Source: CAD feature listing. Evaluate the final solid. Frame: model axes, mm. A direction names the side the tool comes from. Round coordinates to 2 decimals unless told otherwise and drop trailing zeros. Order: outer loops, then holes, each group sorted by start corner. A loop starts at its lowest first (then second) coordinate and runs counter-clockwise, first axis right, second up. Notation, with made-up numbers: (75.5, 57.25) - (103.5, 57.25) arc R20 cw to (103.5, 61.25) - close; hole circle Ø8 at (28, 79). An arc over 180 degrees is marked (long way). Put each result on its own line as item: value. Start each with the question number.
1) Section C-C on x = 0. Output: boundary loops of the cut face in (y, z).
2) Section D-D on z = 1.5. Output: boundary loops of the cut face in (x, y), then the cut area to 3 significant figures.
3) Section B-B on z = 5. Output: boundary loops of the cut face in (x, y).
4) Access query for faces 1 (the face through (1.7, 1.4, 4.9)), 2 (the face through (-1.7, 1.5, 4.9)), 3 (the face through (1.864, -0.314, 7.372)). Directions: +Z, -Z, +X, -X, +Y, -Y. A direction counts if a zero-diameter tool reaches every point of the face in a straight line with its end or side. Return the directions, or none.
5) Contact query for flat-ended pins moving along their axis: P1, Ø1.2, axis at x = 2.5, z = 6, coming from the +Y side; P2, Ø2, axis at y = 0, z = 4.5, coming from the +X side; P3, Ø0.6, axis at y = 1.5, z = 4.5, coming from the -X side; P4, Ø0.9, axis at y = 1.5, z = 6.5, coming from the +X side. Output: stop coordinate, or through.
6) Mould query, pull axis Z, two halves, no side actions, for faces 4 (the face through (0, -1.5, 1)), 5 (the face through (0, 0, 0)), 6 (the face through (-1.3, 0.7, 6.3)). Classes: +Z half, -Z half, draft (parallel to the pull), parting line (faces both ways), or undercut.
7) Section A-A on y = -0.75. Output: boundary loops of the cut face in (x, z).
8) Line query: probe 1 along Z at (x, y) = (-1.3, 0.3); probe 2 along Z at (x, y) = (0, 1.4); probe 3 along Y at (x, z) = (-0.95, 6.5). Output: solid intervals per line, ascending. Write a range as [from, to].
Autodesk Fusion 360 part; units mm, degrees
sketch "Sketch1" plane through (0, 0, 0) normal (0, 0, 1) x (1, 0, 0)
  line L0 (-2.85, 0.9) -> (-2.85, -1.5)
  line L1 (2.85, -1.5) -> (2.85, 0.9)
  line L2 (2.85, 0.9) -> (1.7, 0.9)
  line L3 (1.7, 0.9) -> (1.7, 2)
  line L4 (1.7, 2) -> (-1.7, 2)
  line L5 (-1.7, 2) -> (-1.7, 0.9)
  line L6 (-1.7, 0.9) -> (-2.85, 0.9)
  line L7 (-2.85, -1.5) -> (2.85, -1.5)
  dimension "d1" = 3.4
  dimension "d2" = 5.7
  dimension "d3" = 2.4
  dimension "d4" = 1.1
  dimension "d5" = 1.7
  dimension "d6" = 2
  dimension "d7" = 1.15
extrude "Extrude1" add sketch "Sketch1" along normal blind 10
sketch "Sketch2" plane through (0, -1.5, 0) normal (0, -1, 0) x (1, 0, 0)
  line L0 (-2.85, 0) -> (2.85, 0)
  line L1 (2.85, 0) -> (2.85, 10)
  line L2 (2.85, 10) -> (-2.85, 10)
  line L3 (-2.85, 10) -> (-2.85, 0)
  line L4 (1.6166, 2.2) -> (3.2332, 5)
  line L5 (3.2332, 5) -> (1.6166, 7.8)
  line L6 (1.6166, 7.8) -> (-1.6166, 7.8)
  line L7 (-1.6166, 7.8) -> (-3.2332, 5)
  line L8 (-3.2332, 5) -> (-1.6166, 2.2)
  line L9 (-1.6166, 2.2) -> (1.6166, 2.2)
  circle A0 centre (0, 5) radius 1.5
  point P0 (0, 5)
  dimension "d10" = 2.8
  dimension "d11" = 2.85
  dimension "d19" = 5
  dimension "d20" = 3
extrude "Extrude2" cut sketch "Sketch2" against normal blind 2.2 contours L1 L3 L4 L5 L6 L7 L8 L9 | A0
fillet "Fillet1" radius 0.4 4 edges at (-2.85, -0.4, 4.3363) (2.85, -0.4, 5.6637) (2.85, -0.4, 4.3363) (-2.85, -0.4, 5.6637)
fillet "Fillet2" radius 0.4 8 edges at (-1.7, 1.45, 0) (-2.85, -0.3, 0) (-2.85, -0.3, 10) (-1.7, 1.45, 10) (1.7, 1.45, 0) (2.85, -0.3, 0) (1.7, 1.45, 10) (2.85, -0.3, 10)
chamfer "Chamfer1" distance 0.2 angle 45 20 edges at (0, -1.5, 0) (2.7328, -1.5, 0.1172) (2.85, -1.5, 1.6218) (2.5535, -1.5, 3.2299) (1.8601, -1.5, 2.6218) (-1.8601, -1.5, 2.6218) (-2.5535, -1.5, 3.2299) (-2.85, -1.5, 1.6218) (-2.7328, -1.5, 0.1172) (0, -1.5, 2.2) (-2.85, -1.5, 8.3782) (-2.7328, -1.5, 9.8828) (0, -1.5, 10) (2.7328, -1.5, 9.8828) (2.85, -1.5, 8.3782) (2.5535, -1.5, 6.7701) (1.8601, -1.5, 7.3782) (-1.8601, -1.5, 7.3782) (-2.5535, -1.5, 6.7701) (0, -1.5, 7.8)
extrude "Extrude3" cut sketch "Sketch2" against normal blind 5 contours A0
equation "d5 = ( 3.4 / 2 ) * 1 mm"
equation "d7 = ( ( 5.7 - 3.4 ) / 2 ) * 1 mm"
equation "d10 = ( 5.6 / 2 ) * 1 mm"
equation "d11 = ( 5.7 / 2 ) * 1 mm"
Answer sheet:
1. outline: (-1.5, 0.2) - (-1.3, 0) - (2, 0) - (2, 3.5) - (0.7, 3.5) - (0.7, 2.2) - (-1.3, 2.2) - (-1.5, 2) - close; (-1.5, 8) - (-1.3, 7.8) - (0.7, 7.8) - (0.7, 6.5) - (2, 6.5) - (2, 10) - (-1.3, 10) - (-1.5, 9.8) - close
2. outline: (-2.85, -1.3) - (-2.65, -1.5) - (2.65, -1.5) - (2.85, -1.3) - (2.85, 0.9) - (1.7, 0.9) - (1.7, 2) - (-1.7, 2) - (-1.7, 0.9) - (-2.85, 0.9) - close
2. area: 17.4 mm^2
3. outline: (-2.85, 0.7) - (-1.5, 0.7) - (-1.5, 2) - (-1.7, 2) - (-1.7, 0.9) - (-2.85, 0.9) - close; (1.5, 0.7) - (2.85, 0.7) - (2.85, 0.9) - (1.7, 0.9) - (1.7, 2) - (1.5, 2) - close
4. face 1: +Z, -Z, +X, +Y
4. face 2: +Z, -Z, -X, +Y
4. face 3: -Y
5. P1: y = 0.9
5. P2: x = 2.85
5. P3: x = -1.7
5. P4: x = 1.7
6. face 4: draft
6. face 5: -Z half
6. face 6: undercut
7. outline: (-2.85, 0.4) arc R0.4 ccw to (-2.45, 0) - (2.45, 0) arc R0.4 ccw to (2.85, 0.4) - (2.85, 2.84) arc R0.4 ccw to (2.1, 3.04) - (1.62, 2.2) - (-1.62, 2.2) - (-2.1, 3.04) arc R0.4 ccw to (-2.85, 2.84) - close; (-2.85, 7.16) arc R0.4 ccw to (-2.1, 6.96) - (-1.62, 7.8) - (1.62, 7.8) - (2.1, 6.96) arc R0.4 ccw to (2.85, 7.16) - (2.85, 9.6) arc R0.4 ccw to (2.45, 10) - (-2.45, 10) arc R0.4 ccw to (-2.85, 9.6) - close
8. probe 1: [0, 2.2], [7.8, 10]
8. probe 2: [0, 3.5], [6.5, 10]
8. probe 3: [0.7, 2]
